from build123d import *
from build123d.topology import SkipClean

# Parameters (mm, degrees)
SKETCH1_R            = 3.5
SHAFT_BOSS_DEPTH     = 60
CUT_2X2_KEYWAY_DEPTH = 1.2
SKETCH3_R            = 6
COLLAR_BOSS_DEPTH    = 2
SKETCH4_R            = 4.25
HANDLE_BOSS_DEPTH    = 12
CUT_3X3_KEYWAY_DEPTH = 1.8
CHAMFER1_SIZE        = 0.254


with BuildPart() as part:
    # Sketch1 → Shaft-Boss (new body)
    with BuildSketch(Plane(origin=(0, 0, 0), x_dir=(0, 0, -1), z_dir=(1, 0, 0))):
        Circle(SKETCH1_R)
    extrude(amount=SHAFT_BOSS_DEPTH)

    # Sketch2 → Cut-2x2 Keyway (cut)
    with BuildSketch(Plane(origin=(0, 3.5, 0), x_dir=(-1, 0, 0), z_dir=(0, 1, 0))):
        with BuildLine():
            Line((-25, -1), (-40, -1))
            ThreePointArc((-40, -1), (-41, 0), (-40, 1))
            Line((-40, 1), (-25, 1))
            ThreePointArc((-25, 1), (-24, 0), (-25, -1))
        make_face()
    extrude(amount=-CUT_2X2_KEYWAY_DEPTH, mode=Mode.SUBTRACT)

    # Sketch3 → Collar-Boss (add)
    with BuildSketch(Plane(origin=(60, 0, 0), x_dir=(0, 0, -1), z_dir=(1, 0, 0))):
        Circle(SKETCH3_R)
    extrude(amount=COLLAR_BOSS_DEPTH)

    # Sketch4 → Handle-Boss (add)
    with BuildSketch(Plane(origin=(62, 0, 0), x_dir=(0, 0, -1), z_dir=(1, 0, 0))):
        Circle(SKETCH4_R)
    extrude(amount=HANDLE_BOSS_DEPTH)

    # Sketch5 → Cut-3x3 Keyway (cut)
    with SkipClean():  # the faces are left unmerged after this step: merging them gives an invalid solid
        with BuildSketch(Plane.XY.offset(4.25)):
            with BuildLine():
                Line((83.5, -1.5), (63.5, -1.5))
                ThreePointArc((63.5, -1.5), (62, 0), (63.5, 1.5))
                Line((63.5, 1.5), (83.5, 1.5))
                ThreePointArc((83.5, 1.5), (85, 0), (83.5, -1.5))
            make_face()
        extrude(amount=-CUT_3X3_KEYWAY_DEPTH, mode=Mode.SUBTRACT)

    # Chamfer1
    chamfer1_edges = [part.edges().sort_by_distance(p)[0] for p in [
        (0, 0, 3.5),
        (74, -4.181064283, -0.7623657),
    ]]
    chamfer(chamfer1_edges, length=CHAMFER1_SIZE)


solid = part.part
Geometry check sheet. Reference: the model listing, model coordinates, mm. A direction names the side the tool comes from. Give positions to 0.01 mm unless a question says otherwise; leave off trailing zeros. Loops run counter-clockwise (first coordinate to the right, second up) from the corner with the lowest first, then second, coordinate; pieces in that order, holes last. Notation, with made-up numbers: (75.25, 86.5) -> (95.25, 86.5) arc R28 cw to (95.25, 124.5) -> close; hole circle Ø2 at (27, 67.5). An arc over 180 degrees is marked (long way). Answer in a Markdown table with one row per item. Add a question column.
1) Material ranges on probe 1 along X at (y, z) = (2.75, 0.75); probe 2 along X at (y, z) = (0.5, 5); probe 3 along X at (y, z) = (3.25, -0.25), recorded low to high. Write a range as from..to.
2) Draft check along Z on faces 5 (the face through (62, -4, -3)), 6 (the face through (29.709, -3.417, 0.759)), 7 (the face through (24, 3, 0)), 8 (the face through (68, 0, 2.45)). Enter one of: pulls with the +Z half, pulls with the -Z half, needs draft (parallel to the pull), parting line crosses it, or undercut.
3) Cross-section at A-A on z = 0. Record the boundary of the cut face in (x, y), and give its area (3 significant figures).
4) Gauge pin test, flat ends, axial feed: P1, Ø3, axis at x = 14.5, y = -3, coming from the +Z side; P2, Ø1, axis at x = 16.5, z = 0, coming from the +Y side; P3, Ø5, axis at x = 13.5, y = -4.5, coming from the +Z side. Record the tip position at first contact, or that the pin passes through.
5) Cross-section at C-C on y = 5. Record the boundary of the cut face in (x, z), and give its area (3 significant figures).
6) Cross-section at D-D on x = 54. Record the boundary of the cut face in (y, z).
7) Set-up check for faces 1 (the face through (61, 0, 6)), 2 (the face through (32, 2.3, 0)), 3 (the face through (69, 1.5, 3)), 4 (the face through (60, -3, -3)): record each of +Z, -Z, +X, -X, +Y, -Y from which the full face is reachable in a straight line by a thin tool's end or side.
8) Cross-section at B-B on x = 30. Record the boundary of the cut face in (y, z), and give its area (3 significant figures).
Outcome:
| question | item | result |
|---|---|---|
| 1 | probe 1 | x = 0..24.34, 40.66..74 |
| 1 | probe 2 | x = 60..62 |
| 1 | probe 3 | x = 0.01..24.03, 40.97..74 |
| 2 | face 5 | needs draft |
| 2 | face 6 | parting line crosses it |
| 2 | face 7 | undercut |
| 2 | face 8 | pulls with the +Z half |
| 3 | outline | (0, -3.25) -> (0.25, -3.5) -> (60, -3.5) -> (60, -6) -> (62, -6) -> (62, -4.25) -> (73.75, -4.25) -> (74, -4) -> (74, 4) -> (73.75, 4.25) -> (62, 4.25) -> (62, 6) -> (60, 6) -> (60, 3.5) -> (41, 3.5) -> (41, 2.3) -> (24, 2.3) -> (24, 3.5) -> (0.25, 3.5) -> (0, 3.25) -> close |
| 3 | area | 525 mm^2 |
| 4 | P1 | stops at z = 3.16 |
| 4 | P2 | stops at y = 3.5 |
| 4 | P3 | stops at z = 2.87 |
| 5 | outline | (60, -3.32) -> (62, -3.32) -> (62, 3.32) -> (60, 3.32) -> close |
| 5 | area | 13.3 mm^2 |
| 6 | outline | circle Ø7 at (0, 0) |
| 7 | face 1 | +X, -X |
| 7 | face 2 | +Y |
| 7 | face 3 | +Z, +X |
| 7 | face 4 | -X |
| 8 | outline | (2.3, -1) -> (2.3, 1) -> (3.35, 1) arc R3.5 ccw (long way) to (3.35, -1) -> close |
| 8 | area | 36.2 mm^2 |
